from build123d import *

# Parameters (mm, degrees)
BOSS_EXTRUDE1_DEPTH             = 66
CUT_EXTRUDE1_DEPTH              = 9.653149759
CUT_EXTRUDE2_REACH              = 10.653
F_2_5_2_5_DIAMETER_HOLE1_D      = 2.5
F_2_5_2_5_DIAMETER_HOLE1_DEPTH  = 8
F_2_5_2_5_DIAMETER_HOLE1_TIP    = 0.751075774
TAP_DRILL_FOR_M2X0_4_TAP1_D     = 1.6
TAP_DRILL_FOR_M2X0_4_TAP1_DEPTH = 8
TAP_DRILL_FOR_M2X0_4_TAP1_TIP   = 0.480688495
F_2_5_2_5_DIAMETER_HOLE2_D      = 2.5
F_2_5_2_5_DIAMETER_HOLE2_DEPTH  = 8
F_2_5_2_5_DIAMETER_HOLE2_TIP    = 0.751075774
TAP_DRILL_FOR_M2X0_4_TAP2_D     = 1.6
TAP_DRILL_FOR_M2X0_4_TAP2_DEPTH = 8
TAP_DRILL_FOR_M2X0_4_TAP2_TIP   = 0.480688495


with BuildPart() as part:
    # Sketch1 → Boss-Extrude1 (new body)
    with BuildSketch(Plane(origin=(0, 66, 0), x_dir=(1, 0, 0), z_dir=(0, 1, 0))):
        Polygon((2.999999997, 0.701867841), (-6, -5.599999997), (-6, -9.6), (-0.331046591, -9.6), (-0.331046591, -5.866580498), (4.618700872, -0.916833034), align=None)
    extrude(amount=-BOSS_EXTRUDE1_DEPTH)

    # Sketch2 → Cut-Extrude1 (cut, through all)
    with BuildSketch(Plane(origin=(2.767766953, 0, 2.767766953), x_dir=(0.707106781, 0, -0.707106781), z_dir=(0.707106781, 0, 0.707106781))):
        with BuildLine():
            Line((-0.382384145, 47.599999993), (-2.382384145, 47.599999993))
            ThreePointArc((-2.382384145, 47.599999993), (-3.982384137, 46.000000001), (-2.382384145, 44.400000009))
            Line((-2.382384145, 44.400000009), (-0.382384145, 44.400000009))
            ThreePointArc((-0.382384145, 44.400000009), (1.217615847, 46.000000001), (-0.382384145, 47.599999993))
        make_face()
    extrude(amount=-CUT_EXTRUDE1_DEPTH, mode=Mode.SUBTRACT)

    # Sketch3 → Cut-Extrude2 (cut, up to next)
    with BuildSketch(Plane(origin=(2.767766953, 0, 2.767766953), x_dir=(0.707106781, 0, -0.707106781), z_dir=(0.707106781, 0, 0.707106781)), mode=Mode.PRIVATE) as cut_extrude2_sk1:
        with BuildLine():
            Line((-0.382384145, 21.599999991), (-2.382384145, 21.599999991))
            ThreePointArc((-2.382384145, 21.599999991), (-3.982384137, 19.999999999), (-2.382384145, 18.400000007))
            Line((-2.382384145, 18.400000007), (-0.382384145, 18.400000007))
            ThreePointArc((-0.382384145, 18.400000007), (1.217615847, 19.999999999), (-0.382384145, 21.599999991))
        make_face()
    cut_extrude2_tool1 = extrude(cut_extrude2_sk1.sketch, amount=-CUT_EXTRUDE2_REACH, mode=Mode.PRIVATE) & part.part
    add(cut_extrude2_tool1.solids().sort_by_distance((1.790274, 20, 3.74526))[0], mode=Mode.SUBTRACT)

    # Ø2.5 (2.5) Diameter Hole1
    with Locations(Plane(origin=(0, 0, 0), x_dir=(-1, 0, 0), z_dir=(0, -1, 0))):
        with Locations((3, -7.1)):
            Hole(F_2_5_2_5_DIAMETER_HOLE1_D / 2, depth=F_2_5_2_5_DIAMETER_HOLE1_DEPTH)
            with Locations((0, 0, -(F_2_5_2_5_DIAMETER_HOLE1_DEPTH + F_2_5_2_5_DIAMETER_HOLE1_TIP / 2))):  # 118° drill point
                Cone(0, F_2_5_2_5_DIAMETER_HOLE1_D / 2, F_2_5_2_5_DIAMETER_HOLE1_TIP, mode=Mode.SUBTRACT)

    # Tap Drill for M2x0.4 Tap1
    with Locations(Plane(origin=(0, 0, 0), x_dir=(-1, 0, 0), z_dir=(0, -1, 0))):
        with Locations((0.604004818, -3.897000298)):
            Hole(TAP_DRILL_FOR_M2X0_4_TAP1_D / 2, depth=TAP_DRILL_FOR_M2X0_4_TAP1_DEPTH)
            with Locations((0, 0, -(TAP_DRILL_FOR_M2X0_4_TAP1_DEPTH + TAP_DRILL_FOR_M2X0_4_TAP1_TIP / 2))):  # 118° drill point
                Cone(0, TAP_DRILL_FOR_M2X0_4_TAP1_D / 2, TAP_DRILL_FOR_M2X0_4_TAP1_TIP, mode=Mode.SUBTRACT)

    # Ø2.5 (2.5) Diameter Hole2
    with Locations(Plane(origin=(0, 66, 0), x_dir=(1, 0, 0), z_dir=(0, 1, 0))):
        with Locations((-3, -7.1)):
            Hole(F_2_5_2_5_DIAMETER_HOLE2_D / 2, depth=F_2_5_2_5_DIAMETER_HOLE2_DEPTH)
            with Locations((0, 0, -(F_2_5_2_5_DIAMETER_HOLE2_DEPTH + F_2_5_2_5_DIAMETER_HOLE2_TIP / 2))):  # 118° drill point
                Cone(0, F_2_5_2_5_DIAMETER_HOLE2_D / 2, F_2_5_2_5_DIAMETER_HOLE2_TIP, mode=Mode.SUBTRACT)

    # Tap Drill for M2x0.4 Tap2
    with Locations(Plane(origin=(0, 66, 0), x_dir=(1, 0, 0), z_dir=(0, 1, 0))):
        with Locations((-0.604004818, -3.897000298)):
            Hole(TAP_DRILL_FOR_M2X0_4_TAP2_D / 2, depth=TAP_DRILL_FOR_M2X0_4_TAP2_DEPTH)
            with Locations((0, 0, -(TAP_DRILL_FOR_M2X0_4_TAP2_DEPTH + TAP_DRILL_FOR_M2X0_4_TAP2_TIP / 2))):  # 118° drill point
                Cone(0, TAP_DRILL_FOR_M2X0_4_TAP2_D / 2, TAP_DRILL_FOR_M2X0_4_TAP2_TIP, mode=Mode.SUBTRACT)


solid = part.part
Build history of the part. All positions in model axes, mm. A direction names the side the tool comes from. Coordinates: 2 decimals unless noted, no trailing zeros. Order: outer loops, then holes, each group sorted by start corner. A loop starts at its lowest first (then second) coordinate and runs counter-clockwise, first axis right, second up. Notation, with made-up numbers: (47.5, 29) - (93.5, 29) arc R17 ccw to (93.5, 42) - close; hole circle Ø11 at (22, -32.5). An arc over 180 degrees is marked (long way). Put each result on its own line as item: value.
1. Tool access for faces 1 (the face through (-0.331, 33, 8)), 2 (the face through (1, 47.6, 3)), 3 (the face through (-0.777, 4.056, 4.678)): list every direction of +Z, -Z, +X, -X, +Y, -Y with a clear straight run to the whole face (end or side of a thin tool).
Answer sheet:
face 1: +Z, +X, +Y, -Y
face 2: none
face 3: -Y
2. Saw through at A-A (y = 6.5). Write the cut outline in (x, z), and give its area (3 significant figures).
Answer sheet:
outline: (-6, 5.6) - (3, -0.7) - (4.62, 0.92) - (-0.33, 5.87) - (-0.33, 9.6) - (-6, 9.6) - close; hole circle Ø2.5 at (-3, 7.1); hole circle Ø1.6 at (-0.6, 3.9)
area: 42.1 mm^2
3. Saw through at B-B (z = 9). Write the cut outline in (x, y), and give its area (3 significant figures).
Answer sheet:
outline: (-6, 0) - (-0.33, 0) - (-0.33, 66) - (-6, 66) - close
area: 374 mm^2
4. Pull direction Y, two halves, no side cores. Call faces 4 (the face through (2.646, 19.965, 0.925)), 5 (the face through (2.109, 33.462, 3.426)), 6 (the face through (-0.63, 57.6, 4.03)): pulls with the +Y half, pulls with the -Y half, needs draft (parallel to the pull), parting line crosses it, or undercut.
Answer sheet:
face 4: undercut
face 5: needs draft
face 6: pulls with the +Y half
5. Probe line 1 along Y through (x, z) = (-0.5, 4.75); line 2 along X through (y, z) = (2.75, 7.1); line 3 along Z through (x, y) = (-3, 62). List the from-to ranges inside material, lowest first. Write a range as [from, to].
Answer sheet:
line 1: y = [0, 19.11], [20.89, 45.11], [46.89, 66]
line 2: x = [-6, -4.25], [-1.75, -0.33]
line 3: z = [3.5, 5.85], [8.35, 9.6]
6. Drop flat-ended pins along their axis: P1, Ø1, axis at y = 15.5, z = 4, coming from the +X side; P2, Ø1.5, axis at y = 12, z = 0.5, coming from the -X side; P3, Ø1, axis at x = -1.5, y = 46, coming from the -Z side. Give the stop position or say it passes through.
Answer sheet:
P1: stops at x = 2.04
P2: stops at x = 0.21
P3: stops at z = 3.63
